Design review of the part built by this model. Coordinates are the model's own, in mm. Give positions to 0.01 mm unless a question says otherwise; leave off trailing zeros. Write each loop counter-clockwise with the first axis right and the second up, starting at its lowest first coordinate (ties: lowest second). Pieces come first, ordered by that corner, then holes. Notation, with made-up numbers: (21.5, -2) -> (46.5, -2) arc R31 cw to (46.5, 28) -> close; hole circle Ø11 at (11.5, 67.5). An arc over 180 degrees is marked (long way). Return JSON: item names as keys, results as strings. Group by question number.
from build123d import *

# Parameters (mm, degrees)
SKETCH1_W           = 14
SKETCH1_H           = 7
BOSS_EXTRUDE1_DEPTH = 185
CUT_EXTRUDE1_DEPTH  = 186.660981361
CUT_EXTRUDE2_DEPTH  = 186.660981361


with BuildPart() as part:
    # Sketch1 → Boss-Extrude1 (new body)
    with BuildSketch(Plane.XY):
        with Locations((7, 3.5)):
            Rectangle(SKETCH1_W, SKETCH1_H)
    extrude(amount=BOSS_EXTRUDE1_DEPTH)

    # Sketch2 → Cut-Extrude1 (cut, through all)
    with BuildSketch(Plane(origin=(0, 7, 0), x_dir=(1, 0, 0), z_dir=(0, 1, 0))):
        Polygon((0, 0), (14, -14), (14, 0), align=None)
        Polygon((14, -185), (0, -185), (14, -171), align=None)
    extrude(amount=-CUT_EXTRUDE1_DEPTH, mode=Mode.SUBTRACT)

    # Sketch3 → Cut-Extrude2 (cut, through all)
    with BuildSketch(Plane(origin=(0, 7, 0), x_dir=(1, 0, 0), z_dir=(0, 1, 0))):
        with BuildLine():
            Line((8.272792206, -176.727207794), (5.727207794, -179.272792206))
            ThreePointArc((5.727207794, -179.272792206), (5.727207794, -176.727207794), (8.272792206, -176.727207794))
        make_face()
        with BuildLine():
            Line((5.727207794, -5.727207794), (8.272792206, -8.272792206))
            ThreePointArc((8.272792206, -8.272792206), (5.727207794, -8.272792206), (5.727207794, -5.727207794))
        make_face()
    extrude(amount=-CUT_EXTRUDE2_DEPTH, mode=Mode.SUBTRACT)


solid = part.part
Q1. Take a section at B-B, the plane x = 11.75. Give the boundary of the cut face in (y, z).
Q2. For L1, parallel to Z at x = 1, y = 4.5; L2, parallel to Z at x = 9.5, y = 3; L3, parallel to X at y = 6.5, z = 172.5, list the stretches that pass through material, from the lowest coordinate up. Write a range as from..to.
Q3. Take a section at A-A, the plane y = 2.25. Give the boundary of the cut face in (x, z), plus the area to 3 significant figures.
Q4. Insertion check: pin 1 (1 mm diameter, centred on x = 12, y = 3, fed in from -Z); pin 2 (1 mm diameter, centred on x = 10.5, y = 2.5, fed in from -Z). Each pin has a flat end and moves straight along its axis. Give the tip position at first contact, or say it passes through.
Q5. Take a section at C-C, the plane z = 172.5. Give the boundary of the cut face in (x, y), plus the area to 3 significant figures.
Final values:
{
 "1": {"outline": "(0, 11.75) -> (7, 11.75) -> (7, 173.25) -> (0, 173.25) -> close"},
 "2": {"L1": "z = 1..184", "L2": "z = 9.5..175.5", "L3": "x = 0..12.5"},
 "3": {"outline": "(0, 0) -> (5.73, 5.73) arc R1.8 cw to (8.27, 8.27) -> (14, 14) -> (14, 171) -> (8.27, 176.73) arc R1.8 cw to (5.73, 179.27) -> (0, 185) -> close", "area": "2,380 mm²"},
 "4": {"pin 1": "stops at z = 11.5", "pin 2": "stops at z = 10"},
 "5": {"outline": "(0, 0) -> (12.5, 0) -> (12.5, 7) -> (0, 7) -> close", "area": "87.5 mm²"}
}
